```python
from build123d import *

# Parameters (mm, degrees)
SALIENTE_EXTRUIR1_DEPTH        = 2.7
CROQUIS2_OUTSIDE_W             = 57.324
CROQUIS2_OUTSIDE_H             = 60.248
CROQUIS2_OUTSIDE_R             = 9.25
CORTAR_EXTRUIR1_DEPTH          = 2.7
CORTAR_EXTRUIR1_DRAFT          = -80
CROQUIS3_OUTSIDE_W             = 41.536
CROQUIS3_OUTSIDE_H             = 44.46
CROQUIS3_OUTSIDE_R             = 9.25
CORTAR_EXTRUIR2_DEPTH          = 2.7
CORTAR_EXTRUIR2_DRAFT          = -70
TALADRO_ROSCADO_M16X1_51_D     = 14.5
TALADRO_ROSCADO_M16X1_51_DEPTH = 39.5
TALADRO_ROSCADO_M16X1_51_TIP   = 4.356239488


with BuildPart() as part:
    # Croquis1 → Saliente-Extruir1 (new body)
    with BuildSketch(Plane(origin=(0, 0, 0), x_dir=(1, 0, 0), z_dir=(0, 1, 0))):
        Polygon((0, -10.911920088), (9.45, -5.455960044), (9.45, 5.455960044), (0, 10.911920088), (-9.45, 5.455960044), (-9.45, -5.455960044), align=None)
    extrude(amount=SALIENTE_EXTRUIR1_DEPTH)


with BuildPart() as cortar_extruir1_tool:
    # Croquis2 outside → Cortar-Extruir1 (with draft: the straight prism first)
    with BuildSketch(Plane(origin=(0, 2.7, 0), x_dir=(1, 0, 0), z_dir=(0, 1, 0))):
        Rectangle(CROQUIS2_OUTSIDE_W, CROQUIS2_OUTSIDE_H)
        Circle(CROQUIS2_OUTSIDE_R, mode=Mode.SUBTRACT)
    extrude(amount=-CORTAR_EXTRUIR1_DEPTH)
    # Cortar-Extruir1: the draft: its side faces are tilted about the plane it starts from
    cortar_extruir1_sides = [cortar_extruir1_tool.faces().sort_by_distance(p)[0] for p in [
        (0, 1.35, 30.124),
        (28.662, 1.35, 0),
        (0, 1.35, -30.124),
        (-28.662, 1.35, 0),
        (-9.25, 1.35, 0),
    ]]
    draft(cortar_extruir1_sides, Plane(origin=(0, 2.7, 0), x_dir=(1, 0, 0), z_dir=(0, 1, 0)), CORTAR_EXTRUIR1_DRAFT)


with BuildPart() as part_1:
    add(part.part)

    # Cortar-Extruir1: cut by cortar_extruir1_tool
    add(cortar_extruir1_tool.part, mode=Mode.SUBTRACT)


with BuildPart() as cortar_extruir2_tool:
    # Croquis3 outside → Cortar-Extruir2 (with draft: the straight prism first)
    with BuildSketch(Plane(origin=(0, 0, 0), x_dir=(-1, 0, 0), z_dir=(0, -1, 0))):
        Rectangle(CROQUIS3_OUTSIDE_W, CROQUIS3_OUTSIDE_H)
        Circle(CROQUIS3_OUTSIDE_R, mode=Mode.SUBTRACT)
    extrude(amount=-CORTAR_EXTRUIR2_DEPTH)
    # Cortar-Extruir2: the draft: its side faces are tilted about the plane it starts from
    cortar_extruir2_sides = [cortar_extruir2_tool.faces().sort_by_distance(p)[0] for p in [
        (0, 1.35, 22.23),
        (-20.768, 1.35, 0),
        (0, 1.35, -22.23),
        (20.768, 1.35, 0),
        (9.25, 1.35, 0),
    ]]
    draft(cortar_extruir2_sides, Plane(origin=(0, 0, 0), x_dir=(-1, 0, 0), z_dir=(0, -1, 0)), CORTAR_EXTRUIR2_DRAFT)


with BuildPart() as part_2:
    add(part_1.part)

    # Cortar-Extruir2: cut by cortar_extruir2_tool
    add(cortar_extruir2_tool.part, mode=Mode.SUBTRACT)

    # Taladro roscado M16x1.51
    with Locations(Plane(origin=(0, 2.7, 0), x_dir=(1, 0, 0), z_dir=(0, 1, 0))):
        with Locations((0, 0)):
            Hole(TALADRO_ROSCADO_M16X1_51_D / 2, depth=TALADRO_ROSCADO_M16X1_51_DEPTH)
            with Locations((0, 0, -(TALADRO_ROSCADO_M16X1_51_DEPTH + TALADRO_ROSCADO_M16X1_51_TIP / 2))):  # 118° drill point
                Cone(0, TALADRO_ROSCADO_M16X1_51_D / 2, TALADRO_ROSCADO_M16X1_51_TIP, mode=Mode.SUBTRACT)


solid = part_2.part
```
The listing builds one solid part. Answer for the finished solid, in the listing's coordinates (mm). Coordinates: 2 decimals unless noted, no trailing zeros. Write each loop counter-clockwise with the first axis right and the second up, starting at its lowest first coordinate (ties: lowest second). Pieces come first, ordered by that corner, then holes. Notation, with made-up numbers: M 4.25,66.25 L 41.25,66.25 A28 cw 41.25,91.25 Z; hole C 54,61.25 d8. An arc over 180 degrees is marked long. Use a Markdown table: item, result. Add a question column.
1. Section A-A (z = 0) is taken. Give the vertices of the cut face in (x, y), plus the area to 3 significant figures.
2. Straight lines are drawn through the part: line 1 along X through (y, z) = (2, 2.5); line 2 along X through (y, z) = (1, -0.25); line 3 along Z through (x, y) = (-1, 1.8). For each, find the intervals that lie inside material, in ascending order. Write a range as [from, to].
3. For a pull along X with two mould halves and no side action, classify faces 1 (the flat face through (-9.45, 1, 0)), 2 (the cylindrical face through (-3.35, 1.33, 6.43)), 3 (the flat face through (-6, 2.7, 5)), 4 (the flat face through (4.7, 1.4, 8.2)) as +X half, -X half, draft (parallel to the pull), parting line (faces both ways), or undercut.
4. Given P1, Ø2, axis at x = 6.5, z = -5, coming from the -Y side; P2, Ø1.5, axis at y = 0.5, z = -8.5, coming from the +X side, each flat-ended and moving along its own axis, determine where each tip first touches the part or whether it passes through.
5. Section B-B (y = 1.95) is taken. Give the vertices of the cut face in (x, z), plus the area to 3 significant figures.
Data:
| question | item | result |
|---|---|---|
| 1 | outline | M -9.45,0.07 L -9.25,0 L -7.25,0 L -7.25,2.7 L -9.25,2.7 L -9.45,2.66 Z; M 7.25,0 L 9.25,0 L 9.45,0.07 L 9.45,2.66 L 9.25,2.7 L 7.25,2.7 Z |
| 1 | area | 11.9 mm2 |
| 2 | line 1 | x = [-9.45, -6.81], [6.81, 9.45] |
| 2 | line 2 | x = [-9.45, -7.25], [7.25, 9.45] |
| 2 | line 3 | z = [-10.33, -7.18], [7.18, 10.33] |
| 3 | face 1 | -X half |
| 3 | face 2 | undercut |
| 3 | face 3 | draft |
| 3 | face 4 | +X half |
| 4 | P1 | stops at y = 0 |
| 4 | P2 | stops at x = 5.48 |
| 5 | outline | M -9.45,-5.46 L 0,-10.91 L 9.45,-5.46 L 9.45,5.46 L 0,10.91 L -9.45,5.46 Z; hole C 0,0 d14.5 |
| 5 | area | 144 mm2 |
